Can you work these out from the model? Positions are in its coordinate system, mm. A direction names the side the tool comes from. Give positions to 0.01 mm unless a question says otherwise; leave off trailing zeros. Write each loop counter-clockwise with the first axis right and the second up, starting at its lowest first coordinate (ties: lowest second). Pieces come first, ordered by that corner, then holes. Notation, with made-up numbers: (-17, -3.5) -> (40, -3.5) arc R29 ccw to (40, 16.5) -> close; hole circle Ø8 at (-20, 67.5). An arc over 180 degrees is marked (long way). One line per item, written item: value.
from build123d import *

# Parameters (mm, degrees)
F1_DEPTH      = 10
F2_R          = 1
F3_R          = 1
F4_R          = 1
F5_R          = 1
F6_W          = 4
F6_H          = 15.75
F7_DEPTH      = 10.001
F7_DEPTH_BACK = 10.001
F8_R          = 2


with BuildPart() as f1:
    # F0 (on Front) → F1 (new body)
    with BuildSketch(Plane.XZ):
        with BuildLine():
            Line((-10, 0), (0, 0))
            Line((0, 0), (10, 0))
            Line((10, 0), (10, 2.25))
            Line((10, 2.25), (6.5, 2.25))
            ThreePointArc((6.5, 2.25), (5.0857864376, 2.8357864376), (4.5, 4.25))
            Line((4.5, 4.25), (4.5, 18))
            Line((4.5, 18), (2.5, 18))
            ThreePointArc((2.5, 18), (0.9, 16.4), (2.5, 14.8))
            Line((2.5, 14.8), (2.5, 4))
            ThreePointArc((2.5, 4), (0, 1.5), (-2.5, 4))
            Line((-2.5, 4), (-2.5, 14.8))
            ThreePointArc((-2.5, 14.8), (-0.9, 16.4), (-2.5, 18))
            Line((-2.5, 18), (-4.5, 18))
            Line((-4.5, 18), (-4.5, 4.25))
            ThreePointArc((-4.5, 4.25), (-5.0857864376, 2.8357864376), (-6.5, 2.25))
            Line((-6.5, 2.25), (-10, 2.25))
            Line((-10, 2.25), (-10, 0))
        make_face()
    extrude(amount=F1_DEPTH)

    # F2
    f2_edges = [f1.edges().sort_by_distance(p)[0] for p in [
        (4.5, -5, 18),
    ]]
    fillet(f2_edges, radius=F2_R)

    # F3
    f3_edges = [f1.edges().sort_by_distance(p)[0] for p in [
        (-4.5, -5, 18),
    ]]
    fillet(f3_edges, radius=F3_R)

    # F4
    f4_edges = [f1.edges().sort_by_distance(p)[0] for p in [
        (10, -5, 2.25),
    ]]
    fillet(f4_edges, radius=F4_R)

    # F5
    f5_edges = [f1.edges().sort_by_distance(p)[0] for p in [
        (-10, -5, 2.25),
    ]]
    fillet(f5_edges, radius=F5_R)

    # F6 (on Right) → F7 (cut, two sides)
    with BuildSketch(Plane.YZ) as f7_sk:
        with Locations((-8, 10.125)):
            Rectangle(F6_W, F6_H)
    extrude(amount=-F7_DEPTH, mode=Mode.SUBTRACT)
    extrude(f7_sk.sketch, amount=F7_DEPTH_BACK, mode=Mode.SUBTRACT)

    # F8
    f8_edges = [f1.edges().sort_by_distance(p)[0] for p in [
        (-4.142679, -6, 2.25),
        (4.142679, -6, 2.25),
    ]]
    fillet(f8_edges, radius=F8_R)


solid = f1.part
1) If we section it at D-D (z = 13.25): Write out the boundary of the cut face in (x, y), and give its area (3 significant figures).
Answer list:
outline: (-4.5, -6) -> (-2.5, -6) -> (-2.5, 0) -> (-4.5, 0) -> close; (2.5, -6) -> (4.5, -6) -> (4.5, 0) -> (2.5, 0) -> close
area: 24.0 mm^2
2) We'd pull the mould along Z, two halves only. Please class faces 1 (the face through (3.652, -6.835, 2.624)), 2 (the face through (-3, -6, 11)), 3 (the face through (-0.9, -3, 16.4)): released by +Z, released by -Z, zero draft, split by the parting line, or undercut.
Answer list:
face 1: released by +Z
face 2: zero draft
face 3: undercut
3) If we section it at B-B (y = -4): Write out the boundary of the cut face in (x, z).
Answer list:
outline: (-10, 0) -> (10, 0) -> (10, 1.25) arc R1 ccw to (9, 2.25) -> (6.5, 2.25) arc R2 cw to (4.5, 4.25) -> (4.5, 17) arc R1 ccw to (3.5, 18) -> (2.5, 18) arc R1.6 ccw to (2.5, 14.8) -> (2.5, 4) arc R2.5 cw to (-2.5, 4) -> (-2.5, 14.8) arc R1.6 ccw to (-2.5, 18) -> (-3.5, 18) arc R1 ccw to (-4.5, 17) -> (-4.5, 4.25) arc R2 cw to (-6.5, 2.25) -> (-9, 2.25) arc R1 ccw to (-10, 1.25) -> close
4) For faces 4 (the face through (0.1, -3.8, 1.5)), 5 (the face through (-7, -6, 2.25)), 6 (the face through (3, -6, 11)), 7 (the face through (-10, -5, 1)), 8 (the face through (4.5, -3, 11)), which set-ups out of +Z, -Z, +X, -X, +Y, -Y let a thin tool reach every point of the face, with its end or its side?
Answer list:
face 4: +Y, -Y
face 5: +Z, -X, -Y
face 6: +Z, +X, -X, -Y
face 7: +Z, -Z, -X, +Y, -Y
face 8: +Z, +X, +Y, -Y
5) If we section it at C-C (x = 3.25): Write out the boundary of the cut face in (y, z), and give its area (3 significant figures).
Answer list:
outline: (-10, 0) -> (0, 0) -> (0, 18) -> (-6, 18) -> (-6, 4.25) arc R2 cw to (-8, 2.25) -> (-10, 2.25) -> close
area: 118 mm^2
6) I need wall thicknesses on L1, parallel to X at y = -4.25, z = 8.75; L2, parallel to Y at x = -3, z = 14.25; L3, parallel to Z at x = -9, y = -5.75. Which ranges of each line are inside material? Lowest first, please.
Answer list:
L1: x = -4.5 to -2.5, 2.5 to 4.5
L2: y = -6 to 0
L3: z = 0 to 2.25
7) If we section it at A-A (z = 16.4): Write out the boundary of the cut face in (x, y).
Answer list:
outline: (-4.5, -6) -> (-0.9, -6) -> (-0.9, 0) -> (-4.5, 0) -> close; (0.9, -6) -> (4.5, -6) -> (4.5, 0) -> (0.9, 0) -> close
8) Will these pins go through, and if not, where does the flat tip stop? pin 1 (8 mm diameter, centred on x = -4.5, z = 6.5, fed in from +Y); pin 2 (10 mm diameter, centred on x = 0.5, z = 10.5, fed in from -Y); pin 3 (5 mm diameter, centred on y = -1.5, z = 11, fed in from -X); pin 4 (2 mm diameter, centred on y = -3.5, z = 12, fed in from +X).
Answer list:
pin 1: stops at y = 0
pin 2: stops at y = -6
pin 3: stops at x = -4.5
pin 4: stops at x = 4.5
